The model under review builds one solid part; all positions refer to its coordinate system, in mm. A direction names the side the tool comes from. Give positions to 0.01 mm unless a question says otherwise; leave off trailing zeros. Loops run counter-clockwise (first coordinate to the right, second up) from the corner with the lowest first, then second, coordinate; pieces in that order, holes last. Notation, with made-up numbers: M 43,17 L 49,17 A28 ccw 49,36 Z; hole C 81.5,21.25 d6. An arc over 180 degrees is marked long. Write item = value, one per line. Start each with the question number.
1. We need section C-C on z = 1.25. Give the boundary of the cut face in (x, y), then the cut area to 3 significant figures.
2. Wall thickness on line 1 along Z through (x, y) = (11.75, -1); line 2 along X through (y, z) = (-2, -1.5); line 3 along Z through (x, y) = (2, 3.75): over which ranges is each line inside the solid? List them lowest first. Write a range as from..to.
3. We need section A-A on y = -3.25. Give the boundary of the cut face in (x, z).
4. For pin 1 (1.5 mm diameter, centred on y = 1, z = 9, fed in from +X); pin 2 (4 mm diameter, centred on x = 15.73, y = -2.86, fed in from -Z); pin 3 (2 mm diameter, centred on x = 6, y = -1, fed in from +Z); pin 4 (2.5 mm diameter, centred on x = 8, y = -0.78, fed in from -Z), all flat-tipped, find the tip position at first contact; note any pin that passes through.
5. We need section D-D on x = 8. Give the boundary of the cut face in (y, z), then the cut area to 3 significant figures.
6. For faces 1 (the face through (9.062, 3.072, 7.218)), 2 (the face through (12.86, 3.07, 6.28)), 3 (the face through (20, -2, -10)), 4 (the face through (10.278, 2.746, 13.486)), list the 3-axis set-ups (+Z, -Z, +X, -X, +Y, -Y) from which the entire face can be reached by the end or side of a thin tool; tool diameter is ignored.
7. Draft analysis for pull direction Y (two halves, no side actions). For faces 5 (the face through (2.535, -1.617, -0.177)), 6 (the face through (10, -1, -12.5)), 7 (the face through (10.278, 2.746, -13.514)), state which applies: pulls with the +Y half, pulls with the -Y half, needs draft (parallel to the pull), parting line crosses it, or undercut.
8. We need section B-B on x = 13.25. Give the boundary of the cut face in (y, z) (3 decimals).
from build123d import *

# Parameters (mm, degrees)
SKETCH_1_W          = 25
SKETCH_1_H          = 11
EXTRUDE_1_DEPTH     = 5
SKETCH_2_W          = 4
SKETCH_2_H          = 15
EXTRUDE_2_DEPTH     = 15
SKETCH_4_R          = 1.6
CUT_EXTRUDE_1_DEPTH = 34.395358959
EXTRUDE_3_DEPTH     = 2
CUT_EXTRUDE_2_DEPTH = 37.4451986
SKETCH_8_R          = 3
CUT_EXTRUDE_3_DEPTH = 23.744804244
SKETCH_9_W          = 8
SKETCH_9_H          = 6.263890715
CUT_EXTRUDE_4_DEPTH = 23.744804244
FILLET_1_R          = 3


with BuildPart() as part:
    # 草图1 → 凸台-拉伸1 (new body)
    with BuildSketch(Plane(origin=(0, 0, 0), x_dir=(0, 0, -1), z_dir=(1, 0, 0))):
        Rectangle(SKETCH_1_W, SKETCH_1_H)
    extrude(amount=EXTRUDE_1_DEPTH)

    # 草图2 → 凸台-拉伸2 (add)
    with BuildSketch(Plane(origin=(5, 0, 0), x_dir=(0, 0, -1), z_dir=(1, 0, 0))):
        with Locations((-10.5, -2)):
            Rectangle(SKETCH_2_W, SKETCH_2_H)
        with Locations((10.5, -2)):
            Rectangle(SKETCH_2_W, SKETCH_2_H)
    extrude(amount=EXTRUDE_2_DEPTH)

    # 草图4 → 切除-拉伸1 (cut, through all)
    with BuildSketch(Plane.XY.offset(12.5)):
        with Locations((15.72740661, -2.855250622)):
            Circle(SKETCH_4_R)
        with Locations((8, -0.784698261)):
            Circle(SKETCH_4_R)
        Polygon((0, 5.5), (20, 0.141016151), (20, 5.5), align=None)
        Polygon((0, -2.782209443), (20, -8.141193292), (20, -9.5), (0, -9.5), align=None)
    extrude(amount=-CUT_EXTRUDE_1_DEPTH, mode=Mode.SUBTRACT)

    # 草图6 → 凸台-拉伸3 (add)
    with BuildSketch(Plane(origin=(1.375, 5.13156986, 0), x_dir=(0.96592582628907, -0.25881904510251436, 0), z_dir=(0.25881904510251436, 0.96592582628907, 0))):
        Polygon((19.28201886, 8.5), (19.28201886, 14.5), (-1.423504748, 14.5), (-1.423504748, -14.5), (19.28201886, -14.5), (19.28201886, -8.5), (3.752876154, -4), (3.752876154, 4), align=None)
    extrude(amount=EXTRUDE_3_DEPTH)

    # 草图7 → 切除-拉伸2 (cut, through all)
    with BuildSketch(Plane.XY.offset(14.5)):
        Polygon((1.342544747, 7.21081858), (0, 2.200373372), (-7.179719812, 0.653741147), (-4.482102144, 8.771528011), align=None)
    extrude(amount=-CUT_EXTRUDE_2_DEPTH, mode=Mode.SUBTRACT)

    # 草图8 → 切除-拉伸3 (cut, through all)
    with BuildSketch(Plane(origin=(5, 0, 0), x_dir=(0, 0, -1), z_dir=(1, 0, 0))):
        with Locations(Location((0, 1.378044595, 0), (0, 0, 15.908958728))):
            Circle(SKETCH_8_R)
    extrude(amount=-CUT_EXTRUDE_3_DEPTH, mode=Mode.SUBTRACT)

    # 草图9 → 切除-拉伸4 (cut, through all)
    with BuildSketch(Plane(origin=(5, 0, 0), x_dir=(0, 0, -1), z_dir=(1, 0, 0))):
        with Locations((0, 3.617975326)):
            Rectangle(SKETCH_9_W, SKETCH_9_H)
    extrude(amount=CUT_EXTRUDE_4_DEPTH, mode=Mode.SUBTRACT)

    # 圆角1
    fillet_1_edges = [part.edges().sort_by_distance(p)[0] for p in [
        (20, -8.141193292, 10.5),
        (20, -8.141193292, -10.5),
    ]]
    fillet(fillet_1_edges, radius=FILLET_1_R)


solid = part.part
Final values:
q1.outline = M 0,-2.78 L 5,-4.12 L 5,-1.35 L 0,-1.35 Z; M 0.51,4.11 L 5,4.11 L 5,6.23 L 1.34,7.21 Z
q1.area = 21.4 mm²
q2.line_1 = -12.5..-8.5, 8.5..12.5
q2.line_2 = 0..5
q2.line_3 = -12.5..-1.84, 1.84..12.5
q3.outline = M 1.75,-12.5 L 14.18,-12.5 L 14.18,-8.5 L 5,-8.5 L 5,8.5 L 14.18,8.5 L 14.18,12.5 L 1.75,12.5 Z; M 17.28,-12.5 L 20,-12.5 L 20,-8.5 L 17.28,-8.5 Z; M 17.28,8.5 L 20,8.5 L 20,12.5 L 17.28,12.5 Z
q4.pin_1 = 20.43
q4.pin_2 = -12.5
q4.pin_3 = 12.5
q4.pin_4 = through
q5.outline = M -4.93,-12.5 L -2.38,-12.5 L -2.38,-8.5 L -4.93,-8.5 Z; M -4.93,8.5 L -2.38,8.5 L -2.38,12.5 L -4.93,12.5 Z; M 0.82,-12.5 L 3.36,-12.5 L 3.36,-14.5 L 5.43,-14.5 L 5.43,-4.74 L 3.36,-4.9 L 3.36,-8.5 L 0.82,-8.5 Z; M 0.82,8.5 L 3.36,8.5 L 3.36,4.9 L 5.43,4.74 L 5.43,14.5 L 3.36,14.5 L 3.36,12.5 L 0.82,12.5 Z
q5.area = 80.7 mm²
q6.face_1 = -Y
q6.face_2 = +X, -Y
q6.face_3 = +Z, -Z, +X, -Y
q6.face_4 = +Z, -X, -Y
q7.face_5 = undercut
q7.face_6 = needs draft
q7.face_7 = pulls with the -Y half
q8.outline = M -6.333,-12.5 L 1.95,-12.5 L 1.95,-14.5 L 4.02,-14.5 L 4.02,-6.32 L 1.95,-6.475 L 1.95,-8.5 L -6.333,-8.5 Z; M -6.333,8.5 L 1.95,8.5 L 1.95,6.475 L 4.02,6.32 L 4.02,14.5 L 1.95,14.5 L 1.95,12.5 L -6.333,12.5 Z
